Autodesk Inventor part; units mm, degrees
ref_plane "YZ Plane" through (0, 0, 0) normal (1, 0, 0) x (0, 1, 0)
ref_plane "XZ Plane" through (0, 0, 0) normal (0, 1, 0) x (-1, 0, 0)
ref_plane "XY Plane" through (0, 0, 0) normal (0, 0, 1) x (1, 0, 0)
sketch "Sketch1" plane through (0, 0, 0) normal (0, 0, 1) x (1, 0, 0)
  line L0 (3.5, 2.0207) -> (3.5, -2.0207)
  line L1 (3.5, -2.0207) -> (0, -4.0415)
  line L2 (0, -4.0415) -> (-3.5, -2.0207)
  line L3 (-3.5, -2.0207) -> (-3.5, 2.0207)
  line L4 (-3.5, 2.0207) -> (0, 4.0415)
  line L5 (0, 4.0415) -> (3.5, 2.0207)
  point P0 (0, 0)
  point P1 (0, 0)
  dimension "d0" = 7
extrude "Extrusion1" add sketch "Sketch1" along normal blind 12
sketch "Sketch2" plane through (0, 0, 12) normal (0, 0, 1) x (1, 0, 0)
  circle A0 centre (0, 0) radius 2
  dimension "d3" = 4
extrude "Extrusion2" add sketch "Sketch2" along normal blind 8
sketch "Sketch3" plane through (0, 0, 0) normal (0, 0, -1) x (-1, 0, 0)
  point P0 (0, 0)
  point P1 (0, 0)
hole "Hole1" at (0, 0, 0) direction (0, 0, 1) diameter 3.242 depth 11.8 tip angle 118
chamfer "Chamfer1" distance 0.5 angle 45 1 edges at (-2, 0, 20)
thread "Thread1"
properties part number "Abstandshalter_10mm_M4" material "Stainless Steel"
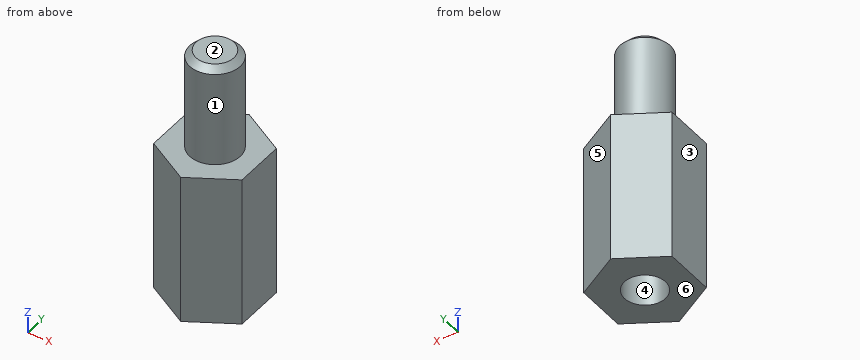
Can you work these out from the model? Positions are in its coordinate system, mm. Face numbers are marked on the shaded views. A direction names the side the tool comes from. Coordinates: 2 decimals unless noted, no trailing zeros. Loops run counter-clockwise (first coordinate to the right, second up) from the corner with the lowest first, then second, coordinate; pieces in that order, holes last. Notation, with made-up numbers: (-29.75, 85) -> (-4.75, 85) arc R26 ccw to (-4.75, 105) -> close; hole circle Ø11 at (56.5, -9). An arc over 180 degrees is marked (long way). Put each result on its own line as item: value. Start each with the question number.
Q1. I want a section at A-A (z = 3.5). Write out the boundary of the cut face in (x, y).
Q2. I'm going to push flat-ended pins straight in: P1, Ø1, axis at y = -2, z = 13, coming from the +X side; P2, Ø1.5, axis at x = 2, z = 11.5, coming from the -Y side. Where does each tip first touch, or does it pass through?
Q3. For the marked faces 1 and 2, which set-ups out of +Z, -Z, +X, -X, +Y, -Y let a thin tool reach every point of the face, with its end or its side?
Q4. I want a section at B-B (z = 18.5). Write out the boundary of the cut face in (x, y).
Q5. If I drill on line 1 (X direction, y = 0, z = 7.25); line 2 (Z direction, x = -0.25, y = -2.25); line 3 (Y direction, x = 0.5, z = 5.5), over which ranges is the centre line in solid material (lowest first)? Write a range as [from, to].
Q6. Thinking about a two-plate mould opening in X: for the marked faces 3, 4, 5 and 6, which applies, pulls with the +X half, pulls with the -X half, needs draft (parallel to the pull), parting line crosses it, or undercut?
Taken from the geometry:
1. outline: (-3.5, -2.02) -> (0, -4.04) -> (3.5, -2.02) -> (3.5, 2.02) -> (0, 4.04) -> (-3.5, 2.02) -> close; hole circle Ø3.24 at (0, 0)
2. P1: stops at x = 1.32
2. P2: stops at y = -3.32
3. face 1: +Z
3. face 2: +Z, +X, -X, +Y, -Y
4. outline: circle Ø4 at (0, 0)
5. line 1: x = [-3.5, -1.62], [1.62, 3.5]
5. line 2: z = [0, 12]
5. line 3: y = [-3.75, -1.54], [1.54, 3.75]
6. face 3: pulls with the -X half
6. face 4: undercut
6. face 5: pulls with the +X half
6. face 6: needs draft
